from build123d import *

# Parameters (mm, degrees)
F0_W         = 3.4
F0_H         = 12.8
F0_W_2       = 8
F0_R         = 1.8
F1_DEPTH     = 45
F2_R         = 1.75
F3_DEPTH     = 25
F2_R_2       = 3
F4_DEPTH     = 2.5
F0_H_2       = 0.6
F5_DEPTH     = 38.2
F6_T3_DEPTH  = 12.8
F6_S4_R      = 1.8
F6_T5_DEPTH  = 8
F6_T8_DEPTH  = 12.8
F6_S9_R      = 1.8
F6_T10_DEPTH = 8
F6_T14_DEPTH = 23.4
F6_T17_DEPTH = 23.4
F6_T20_DEPTH = 23.4
F6_T23_DEPTH = 23.4
F6_T26_DEPTH = 32.8
F6_T29_DEPTH = 32.8
F7_DEPTH     = 41.6


# Not quite as in the source:
# - a fillet or chamfer that OpenCascade refuses, or shapes differently, is made with other operations: its cross-section is extruded or revolved along the edge and cut away or added


with BuildPart() as f1:
    # F0 (on Front) → F1 (new body)
    with BuildSketch(Plane.XZ):
        with Locations((-1.7, 6.4)):
            Rectangle(F0_W, F0_H)
        with Locations((-7.4, 6.4)):
            Rectangle(F0_W_2, F0_H)
        Polygon((-10.8641016151, 6.4), (-9.1320508076, 9.4), (-5.6679491924, 9.4), (-3.9358983849, 6.4), (-5.6679491924, 3.4), (-9.1320508076, 3.4), align=None, mode=Mode.SUBTRACT)
        with Locations((-13.1, 6.4)):
            Rectangle(F0_W, F0_H)
        Polygon((-5.6679491924, 9.4), (-9.1320508076, 9.4), (-10.8641016151, 6.4), (-9.1320508076, 3.4), (-5.6679491924, 3.4), (-3.9358983849, 6.4), align=None)
        with Locations((-7.4, 6.4)):
            Circle(F0_R, mode=Mode.SUBTRACT)
    extrude(amount=F1_DEPTH)

    # F2 (on face) → F3 (cut)
    with BuildSketch(Plane(origin=(-14.8, 0, 0), x_dir=(0, -1, 0), z_dir=(-1, 0, 0))):
        with Locations((5, 6.4)):
            Circle(F2_R)
    extrude(amount=-F3_DEPTH, mode=Mode.SUBTRACT)

    # F2 (on face) → F4 (cut)
    with BuildSketch(Plane(origin=(-14.8, 0, 0), x_dir=(0, -1, 0), z_dir=(-1, 0, 0))):
        with Locations((5, 6.4)):
            Circle(F2_R_2)
        with Locations((5, 6.4)):
            Circle(F2_R, mode=Mode.SUBTRACT)
    extrude(amount=-F4_DEPTH, mode=Mode.SUBTRACT)

    # F0 (on Front) → F5 (cut)
    with BuildSketch(Plane.XZ):
        with Locations((-7.4, 13.1)):
            Rectangle(F0_W_2, F0_H_2)
        with Locations((-7.4, 6.4)):
            Rectangle(F0_W_2, F0_H)
        Polygon((-10.8641016151, 6.4), (-9.1320508076, 9.4), (-5.6679491924, 9.4), (-3.9358983849, 6.4), (-5.6679491924, 3.4), (-9.1320508076, 3.4), align=None, mode=Mode.SUBTRACT)
        with Locations((-7.4, -0.3)):
            Rectangle(F0_W_2, F0_H_2)
        Polygon((-5.6679491924, 9.4), (-9.1320508076, 9.4), (-10.8641016151, 6.4), (-9.1320508076, 3.4), (-5.6679491924, 3.4), (-3.9358983849, 6.4), align=None)
        with Locations((-7.4, 6.4)):
            Circle(F0_R, mode=Mode.SUBTRACT)
    extrude(amount=F5_DEPTH, mode=Mode.SUBTRACT)

    # F6: fillet of radius 4 on 8 edges, made by hand


with BuildPart() as f6_tool1:
    # F6_s2 → F6_t3 (new body)
    with BuildSketch(Plane.XY):
        with BuildLine():
            ThreePointArc((-7.4, -38.2), (-4.5715728753, -37.0284271247), (-3.4, -34.2))
            Line((-3.4, -34.2), (-3.4, -38.2))
            Line((-3.4, -38.2), (-7.4, -38.2))
        make_face()
    extrude(amount=F6_T3_DEPTH)

    # F6_s4 → F6_t5 (cut, symmetric)
    with BuildSketch(Plane.XZ.offset(36.2)):
        with Locations((-7.4, 6.4)):
            Circle(F6_S4_R)
    extrude(amount=F6_T5_DEPTH, both=True, mode=Mode.SUBTRACT)


with BuildPart() as f6_tool6:
    # F6_s7 → F6_t8 (new body)
    with BuildSketch(Plane.XY.offset(12.8)):
        with BuildLine():
            ThreePointArc((-11.4, -34.2), (-10.2284271247, -37.0284271247), (-7.4, -38.2))
            Line((-7.4, -38.2), (-11.4, -38.2))
            Line((-11.4, -38.2), (-11.4, -34.2))
        make_face()
    extrude(amount=-F6_T8_DEPTH)

    # F6_s9 → F6_t10 (cut, symmetric)
    with BuildSketch(Plane.XZ.offset(36.2)):
        with Locations((-7.4, 6.4)):
            Circle(F6_S9_R)
    extrude(amount=F6_T10_DEPTH, both=True, mode=Mode.SUBTRACT)


with BuildPart() as f1_1:
    add(f1.part)

    # F6_t11: union F6_tool1, F6_tool6
    add([f6_tool1.part, f6_tool6.part])


with BuildPart() as f6_tool12:
    # F6_s13 → F6_t14 (new body)
    with BuildSketch(Plane.YZ.offset(10)):
        with BuildLine():
            ThreePointArc((0, 8.8), (-1.1715728753, 11.6284271247), (-4, 12.8))
            Line((-4, 12.8), (0, 12.8))
            Line((0, 12.8), (0, 8.8))
        make_face()
    extrude(amount=-F6_T14_DEPTH)


with BuildPart() as f6_tool15:
    # F6_s16 → F6_t17 (new body)
    with BuildSketch(Plane.YZ.offset(-13.4)):
        with BuildLine():
            ThreePointArc((-4, 0), (-1.1715728753, 1.1715728753), (0, 4))
            Line((0, 4), (0, 0))
            Line((0, 0), (-4, 0))
        make_face()
    extrude(amount=F6_T17_DEPTH)


with BuildPart() as f6_tool18:
    # F6_s19 → F6_t20 (new body)
    with BuildSketch(Plane.YZ.offset(-24.8)):
        with BuildLine():
            ThreePointArc((-4, 0), (-1.1715728753, 1.1715728753), (0, 4))
            Line((0, 4), (0, 0))
            Line((0, 0), (-4, 0))
        make_face()
    extrude(amount=F6_T20_DEPTH)


with BuildPart() as f6_tool21:
    # F6_s22 → F6_t23 (new body)
    with BuildSketch(Plane.YZ.offset(-1.4)):
        with BuildLine():
            ThreePointArc((-4, 12.8), (-1.1715728753, 11.6284271247), (0, 8.8))
            Line((0, 8.8), (0, 12.8))
            Line((0, 12.8), (-4, 12.8))
        make_face()
    extrude(amount=-F6_T23_DEPTH)


with BuildPart() as f6_tool24:
    # F6_s25 → F6_t26 (new body)
    with BuildSketch(Plane.XY.offset(22.8)):
        with BuildLine():
            ThreePointArc((-10.8, -45), (-13.6284271247, -43.8284271247), (-14.8, -41))
            Line((-14.8, -41), (-14.8, -45))
            Line((-14.8, -45), (-10.8, -45))
        make_face()
    extrude(amount=-F6_T26_DEPTH)


with BuildPart() as f6_tool27:
    # F6_s28 → F6_t29 (new body)
    with BuildSketch(Plane.XY.offset(-10)):
        with BuildLine():
            ThreePointArc((0, -41), (-1.1715728753, -43.8284271247), (-4, -45))
            Line((-4, -45), (0, -45))
            Line((0, -45), (0, -41))
        make_face()
    extrude(amount=F6_T29_DEPTH)


with BuildPart() as f1_2:
    add(f1_1.part)

    # F6_t30: cut F6_tool12, F6_tool15, F6_tool18, F6_tool21, F6_tool24, F6_tool27
    add([f6_tool12.part, f6_tool15.part, f6_tool18.part, f6_tool21.part, f6_tool24.part, f6_tool27.part], mode=Mode.SUBTRACT)

    # F0 (on Front) → F7 (cut)
    with BuildSketch(Plane.XZ):
        Polygon((-5.6679491924, 9.4), (-9.1320508076, 9.4), (-10.8641016151, 6.4), (-9.1320508076, 3.4), (-5.6679491924, 3.4), (-3.9358983849, 6.4), align=None)
        with Locations((-7.4, 6.4)):
            Circle(F0_R, mode=Mode.SUBTRACT)
    extrude(amount=F7_DEPTH, mode=Mode.SUBTRACT)


solid = f1_2.part
Here's how the part is built. I have some questions about the finished solid (model axes, mm). A direction names the side the tool comes from. Round coordinates to 2 decimals unless told otherwise and drop trailing zeros. Order: outer loops, then holes, each group sorted by start corner. A loop starts at its lowest first (then second) coordinate and runs counter-clockwise, first axis right, second up. Notation, with made-up numbers: (6.5, -30) -> (26.5, -30) arc R30 ccw to (26.5, 1) -> close; hole circle Ø7 at (-0.5, 34.5). An arc over 180 degrees is marked (long way). Return JSON: item names as keys, results as strings.
Q1. I need wall thicknesses on line 1 along Z through (x, y) = (-13.1, -5); line 2 along X through (y, z) = (-29, 10.75); line 3 along Z through (x, y) = (-1.65, -5). Which ranges of each line are inside material? Lowest first, please. Write a range as from..to.
Filled sheet:
{"line 1": "z = 0..3.4, 9.4..12.8", "line 2": "x = -14.8..-11.4, -3.4..0", "line 3": "z = 0..4.65, 8.15..12.8"}
Q2. Which directions (+Z, -Z, +X, -X, +Y, -Y) give clear straight access to the entire face, cutting with the end or side of a thin tool? Please do faces 4 (the cylindrical face through (-11.86, -3.25, 6.48)), 5 (the flat face through (-3.4, -17, 6)), 6 (the flat face through (-4.8, -39.5, 4.9)).
Filled sheet:
{"face 4": "+X, -X", "face 5": "+Z, -Z, +Y", "face 6": "+Y"}
Q3. If we section it at B-B on y = -32: List the corners of the cut face in (x, z) for me, plus the area to 3 significant figures.
Filled sheet:
{"outline": "(-14.8, 0) -> (-11.4, 0) -> (-11.4, 12.8) -> (-14.8, 12.8) -> close; (-3.4, 0) -> (0, 0) -> (0, 12.8) -> (-3.4, 12.8) -> close", "area": "87.0 mm^2"}
Q4. If we section it at A-A on y = -5: List the corners of the cut face in (x, z) for me.
Filled sheet:
{"outline": "(-14.8, 0) -> (-11.4, 0) -> (-11.4, 4.65) -> (-12.3, 4.65) -> (-12.3, 3.4) -> (-14.8, 3.4) -> close; (-14.8, 9.4) -> (-12.3, 9.4) -> (-12.3, 8.15) -> (-11.4, 8.15) -> (-11.4, 12.8) -> (-14.8, 12.8) -> close; (-3.4, 0) -> (0, 0) -> (0, 4.65) -> (-3.4, 4.65) -> close; (-3.4, 8.15) -> (0, 8.15) -> (0, 12.8) -> (-3.4, 12.8) -> close"}
Q5. For pin 1 Ø2 at (x, y) = (-3.5, -21.5) entering from +Z; pin 2 Ø5 at (x, z) = (-7, 10) entering from +Y (3 decimals), each with a flat end and sliding along its axis, tell me the tip position at first contact or that it passes through.
Filled sheet:
{"pin 1": "stops at z = 12.8", "pin 2": "stops at y = -36.955"}
Q6. If we mould it in two halves opening along Z, with no side actions, what happens to faces 1 (the cylindrical face through (-13.124, -1.203, 1.141)), 2 (the flat face through (-14.8, -20, 6)), 3 (the flat face through (-10, -39.5, 7.9))? For each: released by +Z, released by -Z, zero draft, split by the parting line, or undercut.
Filled sheet:
{"face 1": "released by -Z", "face 2": "zero draft", "face 3": "undercut"}
Q7. If we section it at D-D on z = 11: List the corners of the cut face in (x, y) for me.
Filled sheet:
{"outline": "(-14.8, -41) arc R4 ccw to (-10.8, -45) -> (-4, -45) arc R4 ccw to (0, -41) -> (0, -0.66) -> (-3.4, -0.66) -> (-3.4, -34.2) arc R4 cw to (-11.4, -34.2) -> (-11.4, -0.66) -> (-14.8, -0.66) -> close"}
Q8. If we section it at C-C on x = -13.5: List the corners of the cut face in (y, z) for me.
Filled sheet:
{"outline": "(-43.95, 0) -> (-4, 0) arc R4 ccw to (0, 4) -> (0, 8.8) arc R4 ccw to (-4, 12.8) -> (-43.95, 12.8) -> close; hole circle Ø6 at (-5, 6.4)"}
